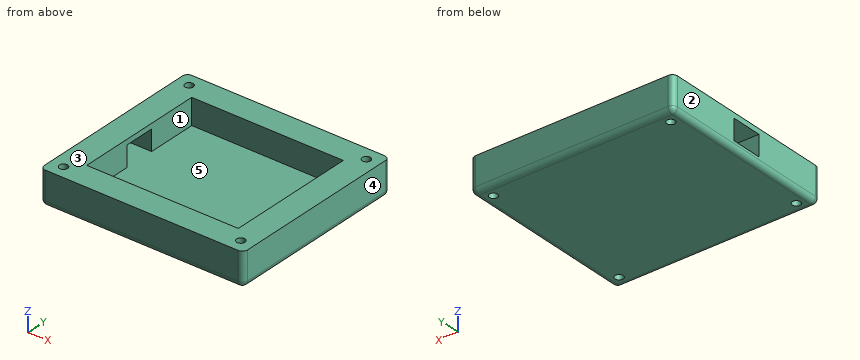
Autodesk Fusion 360 part; units mm, degrees
sketch "Sketch1" plane through (0, 0, 0) normal (0, 0, 1) x (1, 0, 0)
  line L0 (29.4, 25.4) -> (-29.4, 25.4)
  line L1 (-29.4, 25.4) -> (-29.4, -25.4)
  line L2 (-29.4, -25.4) -> (29.4, -25.4)
  line L3 (29.4, -25.4) -> (29.4, 25.4)
  line L4 (29.4, 25.4) -> (-29.4, -25.4) construction
  line L5 (-29.4, 25.4) -> (29.4, -25.4) construction
  line L6 (-39.4, 35.4) -> (-39.4, -35.4)
  line L7 (-39.4, -35.4) -> (39.4, -35.4)
  line L8 (39.4, -35.4) -> (39.4, 35.4)
  line L9 (39.4, 35.4) -> (-39.4, 35.4)
  dimension "d1" = 58.8
  dimension "d2" = 50.8
  dimension "d3" = 10
extrude "Extrude6" add sketch "Sketch1" along normal blind 3 contours L0 L1 L2 L3
extrude "Extrude7" add sketch "Sketch1" along normal blind 13
sketch "Sketch2" plane through (39.4, 0, 0) normal (1, 0, 0) x (0, 1, 0)
  line L0 (-35.4, 0) -> (35.4, 0)
  line L1 (35.4, 0) -> (35.4, 13)
  line L2 (35.4, 13) -> (-35.4, 13)
  line L3 (-35.4, 13) -> (-35.4, 0)
  line L4 (6, 11.3977) -> (-6, 11.3977)
  line L5 (-6, 11.3977) -> (-6, 3.3977)
  line L6 (-6, 3.3977) -> (6, 3.3977)
  line L7 (6, 3.3977) -> (6, 11.3977)
  line L8 (6, 11.3977) -> (-6, 3.3977) construction
  line L9 (-6, 11.3977) -> (6, 3.3977) construction
  point P0 (0, 7.3977)
  dimension "d18" = 12
  dimension "d19" = 8
sketch "Sketch3" plane through (0, 0, 13) normal (0, 0, 1) x (1, 0, 0)
  line L0 (29.4, 25.4) -> (29.4, -25.4)
  line L1 (29.4, -25.4) -> (-29.4, -25.4)
  line L2 (-29.4, -25.4) -> (-29.4, 25.4)
  line L3 (-29.4, 25.4) -> (29.4, 25.4)
  line L4 (39.4, 35.4) -> (-39.4, 35.4)
  line L5 (-39.4, 35.4) -> (-39.4, -35.4)
  line L6 (-39.4, -35.4) -> (39.4, -35.4)
  line L7 (39.4, -35.4) -> (39.4, 35.4)
  circle A0 centre (-34.4, 30.4) radius 1.6
  circle A1 centre (34.4, 30.4) radius 1.6
  circle A2 centre (-34.4, -30.4) radius 1.6
  circle A3 centre (34.4, -30.4) radius 1.6
extrude "Extrude9" cut sketch "Sketch3" against normal blind 13 contours A0 | A1 | A2 | A3
fillet "Fillet1" radius 2 8 edges at (39.4, 0, 0) (39.4, 35.4, 6.5) (39.4, -35.4, 6.5) (0, -35.4, 0) (-39.4, -35.4, 6.5) (-39.4, 0, 0) (-39.4, 35.4, 6.5) (0, 35.4, 0)
sketch "Sketch4" plane through (-39.4, 0, 0) normal (-1, 0, 0) x (0, -1, 0)
  line L0 (-33.4, 13) -> (-33.4, 2)
  line L1 (-33.4, 2) -> (33.4, 2)
  line L2 (33.4, 2) -> (33.4, 13)
  line L3 (33.4, 13) -> (-33.4, 13)
  line L4 (-6, 3.4) -> (6, 3.4)
  line L5 (6, 3.4) -> (6, 11.4)
  line L6 (6, 11.4) -> (-6, 11.4)
  line L7 (-6, 11.4) -> (-6, 3.4)
extrude "Extrude10" cut sketch "Sketch4" along normal blind 10 contours L4 L5 L6 L7
sketch "Sketch5" plane through (39.4, 0, 0) normal (1, 0, 0) x (0, 1, 0)
  line L0 (33.4, 2) -> (33.4, 13)
  line L1 (33.4, 13) -> (-33.4, 13)
  line L2 (-33.4, 13) -> (-33.4, 2)
  line L3 (-33.4, 2) -> (33.4, 2)
  line L4 (-6, 11) -> (6, 11)
  line L5 (6, 11) -> (6, 3)
  line L6 (6, 3) -> (-6, 3)
  line L7 (-6, 3) -> (-6, 11)
  line L8 (-6, 11) -> (6, 3) construction
  line L9 (6, 11) -> (-6, 3) construction
  point P0 (0, 7)
  dimension "d28" = 12
  dimension "d29" = 8
sketch "Sketch6" plane through (0, 0, 0) normal (1, 0, 0) x (0, 1, 0)
sketch "Sketch7" plane through (-39.4, 0, 0) normal (-1, 0, 0) x (0, -1, 0)
  line L0 (-33.4, 13) -> (-33.4, 2)
  line L1 (-33.4, 2) -> (33.4, 2)
  line L2 (33.4, 2) -> (33.4, 13)
  line L3 (33.4, 13) -> (-33.4, 13)
  line L4 (-6, 11) -> (6, 11)
  line L5 (6, 11) -> (6, 3)
  line L6 (6, 3) -> (-6, 3)
  line L7 (-6, 3) -> (-6, 11)
  line L8 (-6, 11) -> (6, 3) construction
  line L9 (6, 11) -> (-6, 3) construction
  point P0 (0, 7)
  dimension "d32" = 12
  dimension "d33" = 8
extrude "Extrude12" cut sketch "Sketch7" against normal blind 27 contours L4 L5 L6 L7
Verification items for the finished model (mm, model axes). Face numbers are marked on the shaded views. A direction names the side the tool comes from. Coordinates: 2 decimals unless noted, no trailing zeros. Loops run counter-clockwise (first coordinate to the right, second up) from the corner with the lowest first, then second, coordinate; pieces in that order, holes last. Notation, with made-up numbers: (-40, 15) -> (5, 15) arc R26 cw to (5, 41) -> close; hole circle Ø6 at (7, 28.25). An arc over 180 degrees is marked (long way). Answer in a Markdown table with one row per item. Add a question column.
1. Section check D-D, the plane x = 34.4. Enter the section's corners in (y, z), then the cut area to 3 significant figures.
2. Depth check by flat-ended pin: P1, Ø5, axis at x = 15, y = -1, coming from the +Z side. Enter the tip coordinate at first touch or a pass-through.
3. Material ranges on probe 1 along Y at (x, z) = (34.4, 5); probe 2 along Y at (x, z) = (-34.4, 9.5); probe 3 along Y at (x, z) = (18.5, 9.75), recorded low to high. Write a range as [from, to].
4. Section check B-B, the plane y = -30.4. Enter the section's corners in (x, z).
5. Section check C-C, the plane y = -2.5. Enter the section's corners in (x, z).
6. Draft check along X on the marked faces 3, 4 and 5. Enter one of: +X half, -X half, draft (parallel to the pull), parting line (faces both ways), or undercut.
7. Section check A-A, the plane x = -34.4. Enter the section's corners in (y, z), then the cut area to 3 significant figures.
8. Access from +Z, -Z, +X, -X, +Y, -Y to the whole of each face (thin tool, end or side, straight path). Record for the marked faces 1 and 2.
Derived:
| question | item | result |
|---|---|---|
| 1 | outline | (-35.4, 2) arc R2 ccw to (-33.4, 0) -> (-32, 0) -> (-32, 13) -> (-35.4, 13) -> close; (-28.8, 0) -> (28.8, 0) -> (28.8, 13) -> (-28.8, 13) -> close; (32, 0) -> (33.4, 0) arc R2 ccw to (35.4, 2) -> (35.4, 13) -> (32, 13) -> close |
| 1 | area | 835 mm² |
| 2 | P1 | stops at z = 3 |
| 3 | probe 1 | y = [-35.4, -32], [-28.8, 28.8], [32, 35.4] |
| 3 | probe 2 | y = [-35.4, -32], [-28.8, -6], [6, 28.8], [32, 35.4] |
| 3 | probe 3 | y = [-35.4, -25.4], [25.4, 35.4] |
| 4 | outline | (-39.4, 2) arc R2 ccw to (-37.4, 0) -> (-36, 0) -> (-36, 13) -> (-39.4, 13) -> close; (-32.8, 0) -> (32.8, 0) -> (32.8, 13) -> (-32.8, 13) -> close; (36, 0) -> (37.4, 0) arc R2 ccw to (39.4, 2) -> (39.4, 13) -> (36, 13) -> close |
| 5 | outline | (-39.4, 2) arc R2 ccw to (-37.4, 0) -> (37.4, 0) arc R2 ccw to (39.4, 2) -> (39.4, 13) -> (29.4, 13) -> (29.4, 3) -> (-39.4, 3) -> close; (-39.4, 11) -> (-29.4, 11) -> (-29.4, 13) -> (-39.4, 13) -> close |
| 6 | face 3 | draft |
| 6 | face 4 | +X half |
| 6 | face 5 | undercut |
| 7 | outline | (-35.4, 2) arc R2 ccw to (-33.4, 0) -> (-32, 0) -> (-32, 13) -> (-35.4, 13) -> close; (-28.8, 0) -> (28.8, 0) -> (28.8, 13) -> (-28.8, 13) -> close; (32, 0) -> (33.4, 0) arc R2 ccw to (35.4, 2) -> (35.4, 13) -> (32, 13) -> close; hole (-6, 3) -> (6, 3) -> (6, 11) -> (-6, 11) -> close |
| 7 | area | 739 mm² |
| 8 | face 1 | +Z |
| 8 | face 2 | +Z, -Z, -X, +Y, -Y |
